from build123d import *

# Parameters (mm, degrees)
F1_DEPTH = 10
F2_R     = 8
F3_DEPTH = 10.001
F4_W     = 14.3
F4_H     = 4.7
F5_DEPTH = 37
F6_W     = 2
F6_H     = 10
F7_DEPTH = 8


with BuildPart() as f1:
    # F0 (on Top) → F1 (new body)
    with BuildSketch(Plane.XY):
        with BuildLine():
            Line((9.15, 0), (9.15, 37.5))
            ThreePointArc((9.15, 37.5), (0, 57.263859), (-9.15, 37.5))
            Line((-9.15, 37.5), (-9.15, 0))
            Line((-9.15, 0), (9.15, 0))
        make_face()
    extrude(amount=F1_DEPTH)

    # F2 (on face) → F3 (cut, through all)
    with BuildSketch(Plane.XY.offset(10)):
        with Locations((0, 45.263859)):
            Circle(F2_R)
    extrude(amount=-F3_DEPTH, mode=Mode.SUBTRACT)

    # F4 (on face) → F5 (cut)
    with BuildSketch(Plane.XZ):
        with Locations((0, 5)):
            Rectangle(F4_W, F4_H)
    extrude(amount=-F5_DEPTH, mode=Mode.SUBTRACT)

    # F6 (on face) → F7 (join)
    with BuildSketch(Plane(origin=(-9.15, 0, 0), x_dir=(0, -1, 0), z_dir=(-1, 0, 0))):
        with Locations((-1, 5)):
            Rectangle(F6_W, F6_H)
        with Locations((-5, 5)):
            Rectangle(F6_W, F6_H)
        with Locations((-11, 5)):
            Rectangle(F6_W, F6_H)
        with Locations((-15, 5)):
            Rectangle(F6_W, F6_H)
    extrude(amount=F7_DEPTH)


solid = f1.part
Can you work these out from the model? Positions are in its coordinate system, mm. A direction names the side the tool comes from. Give positions to 0.01 mm unless a question says otherwise; leave off trailing zeros. Order: outer loops, then holes, each group sorted by start corner. A loop starts at its lowest first (then second) coordinate and runs counter-clockwise, first axis right, second up. Notation, with made-up numbers: M 75,26 L 89,26 A22 ccw 89,42 Z; hole C -23.75,65 d8. An arc over 180 degrees is marked long. Use one line per item in the form item = value.
Item 1: Thinking about a two-plate mould opening in Y: for faces 1 (the flat face through (0, 18, 2.65)), 2 (the flat face through (0, 37, 5)), 3 (the flat face through (-13, 4, 5)), which applies, pulls with the +Y half, pulls with the -Y half, needs draft (parallel to the pull), parting line crosses it, or undercut?
Values follow:
face_1 = needs draft
face_2 = pulls with the -Y half
face_3 = undercut
Item 2: If we section it at C-C, the plane x = 0: Write out the boundary of the cut face in (y, z), and give its area (3 significant figures).
Values follow:
outline = M 0,0 L 37.26,0 L 37.26,10 L 0,10 L 0,7.35 L 37,7.35 L 37,2.65 L 0,2.65 Z; M 53.26,0 L 57.26,0 L 57.26,10 L 53.26,10 Z
area = 239 mm^2
Item 3: If we section it at D-D, the plane z = 1: Write out the boundary of the cut face in (x, y).
Values follow:
outline = M -17.15,0 L 9.15,0 L 9.15,37.5 A12 ccw long -9.15,37.5 L -9.15,16 L -17.15,16 L -17.15,14 L -9.15,14 L -9.15,12 L -17.15,12 L -17.15,10 L -9.15,10 L -9.15,6 L -17.15,6 L -17.15,4 L -9.15,4 L -9.15,2 L -17.15,2 Z; hole C 0,45.26 d16
Item 4: If I drill on line 1 along Y through (x, z) = (0, 2.5); line 2 along Z through (x, y) = (-1.25, 30.5); line 3 along X through (y, z) = (35.5, 3.5), over which ranges is the centre line in solid material (lowest first)? Write a range as [from, to].
Values follow:
line_1 = [0, 37.26], [53.26, 57.26]
line_2 = [0, 2.65], [7.35, 10]
line_3 = [-9.15, -7.15], [7.15, 9.15]
Item 5: Will these pins go through, and if not, where does the flat tip stop? pin 1 Ø5 at (y, z) = (31, 5.5) entering from -X; pin 2 Ø8 at (x, y) = (-13, 9) entering from +Z; pin 3 Ø6 at (y, z) = (41.5, 1.5) entering from -X; pin 4 Ø5 at (y, z) = (15.5, 7) entering from +X.
Values follow:
pin_1 = -9.15
pin_2 = 10
pin_3 = -11.98
pin_4 = 9.15
Item 6: If we section it at B-B, the plane y = 47.5: Write out the boundary of the cut face in (x, z), and give its area (3 significant figures).
Values follow:
outline = M -11.79,0 L -7.68,0 L -7.68,10 L -11.79,10 Z; M 7.68,0 L 11.79,0 L 11.79,10 L 7.68,10 Z
area = 82.2 mm^2
Item 7: For faces 4 (the flat face through (-13, 2, 5)), 5 (the flat face through (-7.15, 18, 5)), 6 (the flat face through (9.15, 18, 5)), which set-ups out of +Z, -Z, +X, -X, +Y, -Y let a thin tool reach every point of the face, with its end or its side?
Values follow:
face_4 = +Z, -Z, -X
face_5 = -Y
face_6 = +Z, -Z, +X, -Y
Item 8: If we section it at A-A, the plane x = -15: Write out the boundary of the cut face in (y, z), and give its area (3 significant figures).
Values follow:
outline = M 0,0 L 2,0 L 2,10 L 0,10 Z; M 4,0 L 6,0 L 6,10 L 4,10 Z; M 10,0 L 12,0 L 12,10 L 10,10 Z; M 14,0 L 16,0 L 16,10 L 14,10 Z
area = 80.0 mm^2
